Source: CAD feature listing. Evaluate the final solid. Frame: model axes, mm. A direction names the side the tool comes from. Round coordinates to 2 decimals unless told otherwise and drop trailing zeros. Order: outer loops, then holes, each group sorted by start corner. A loop starts at its lowest first (then second) coordinate and runs counter-clockwise, first axis right, second up. Notation, with made-up numbers: M -37.75,16 L 3.25,16 A25 cw 3.25,30 Z; hole C -9.5,53.5 d5. An arc over 180 degrees is marked long. Use one line per item in the form item = value. Start each with the question number.
Q1. Reachability of faces 1 (the flat face through (40.488, 0, -4)), 2 (the cylindrical face through (32.51, 9.78, 3.08)), 3 (the cylindrical face through (3.8, -1.72, -7.75)), 4 (the cylindrical face through (11.52, -1.71, -7.72)) from +Z, -Z, +X, -X, +Y, -Y: full face, straight path, thin tool, end or side. Return the list, or none.
Q2. Section B-B (y = 0). Give the number of separate pieces and of enclosed holes in the cut face, plus the area to 3 significant figures.
Q3. Pull-direction query (Z, two-part tool) for faces 5 (the cylindrical face through (34.648, -1.931, -8.697)), 6 (the cylindrical face through (8.797, 6.523, 2.054)), 7 (the conical face through (19.68, 0.06, 10.43)); classes: pulls with the +Z half, pulls with the -Z half, needs draft (parallel to the pull), parting line crosses it, or undercut.
Q4. Contact query for flat-ended pins moving along their axis: pin 1 (10 mm diameter, centred on y = -8, z = 0.5, fed in from -X); pin 2 (12 mm diameter, centred on x = 25, y = 7.5, fed in from +Z); pin 3 (10 mm diameter, centred on x = 24.61, y = 0, fed in from +Z); pin 4 (2 mm diameter, centred on y = 7, z = 5.5, fed in from -X). Output: stop coordinate, or through.
Q5. Section A-A (x = 9). Return the cut outline in (y, z).
Q6. Material intervals for probe 1 along Z at (x, y) = (11.5, 0); probe 2 along X at (y, z) = (7.5, 3.5); probe 3 along Z at (x, y) = (14.5, 0), sorted ascending.
Autodesk Inventor part; units mm, degrees
ref_plane "s1_XY" through (10.3124, 0, 0) normal (0, 0, 1) x (1, 0, 0)
ref_plane "s1_YZ" through (10.3124, 0, 0) normal (1, 0, 0) x (0, 1, 0)
ref_plane "s1_ZX" through (10.3124, 0, 0) normal (0, 1, 0) x (0, 0, 1)
sketch "Sketch_2" plane through (0, 0, 0) normal (0, 0, 1) x (1, 0, 0)
  line L0 (12.7, 0) -> (0, 0)
  line L1 (0, 0) -> (0, 7.098)
  line L2 (0, 7.098) -> (0.8395, 7.9375)
  line L3 (0.8395, 7.9375) -> (6.6816, 7.9375)
  line L4 (6.6816, 7.9375) -> (7.5223, 7.0968)
  arc A0 (7.5223, 7.0968) -> (8.1407, 6.839) centre (8.1385, 7.7041) ccw
  line L5 (8.1407, 6.839) -> (9.4361, 6.839)
  arc A1 (9.4361, 6.839) -> (10.3124, 7.7153) centre (9.4361, 7.7152) ccw
  line L6 (10.3124, 7.7153) -> (10.3124, 7.9057)
  line L7 (10.3124, 7.9057) -> (12.7, 7.9057)
  line L8 (12.7, 7.9057) -> (12.7, 0)
  line L9 (12.7, 0) -> (0, 0)
revolve "Revolution1" add sketch "Sketch_2" angle 360 about axis through (12.7, 0, 0) along (1, 0, 0)
thread "Thread1"
sketch "Sketch_3" plane through (0, 0, 0) normal (0, 0, 1) x (1, 0, 0)
  line L0 (40.4876, 0) -> (12.7, 0)
  line L1 (12.7, 0) -> (12.7, 10.1918)
  line L2 (12.7, 10.1918) -> (13.462, 10.9537)
  line L3 (13.462, 10.9537) -> (34.0741, 10.9537)
  line L4 (34.0741, 10.9537) -> (34.0741, 8.9091)
  line L5 (34.0741, 8.9091) -> (34.8361, 8.9091)
  line L6 (34.8361, 8.9091) -> (35.5981, 9.671)
  line L7 (35.5981, 9.671) -> (39.7256, 9.671)
  line L8 (39.7256, 9.671) -> (40.4876, 8.9091)
  line L9 (40.4876, 8.9091) -> (40.4876, 0)
  line L10 (40.4876, 0) -> (12.7, 0)
revolve "Revolution2" add sketch "Sketch_3" angle 360 about axis through (40.4876, 0, 0) along (1, 0, 0)
sketch "Sketch3" plane through (0, 0, 0) normal (-1, 0, 0) x (0, 0, 1)
  point P0 (0, 0)
hole "Drilling 1" at (0, 0, 0) direction (1, 0, 0) diameter 6.4389 depth 40.4876 countersink diameter 6.9469 countersink angle 90
sketch "Sketch_10" plane through (0, 0, 0) normal (0, 0, 1) x (1, 0, 0)
  line L0 (34.0741, 0) -> (30.8991, 0)
  line L1 (30.8991, 10.2553) -> (34.0741, 10.2553)
  line L2 (34.0741, 10.2553) -> (34.0741, 15.3353)
  line L3 (34.0741, 15.3353) -> (30.8991, 15.3353)
  line L4 (30.8991, 15.3353) -> (30.8991, 10.2553)
revolve "Revolution3" cut sketch "Sketch_10" angle 360 about axis through (34.0741, 0, 0) along (1, 0, 0)
sketch "Sketch_40" plane through (0, 0, 0) normal (0, 1, 0) x (-1, 0, 0)
  line L0 (-24.6126, 10.9537) -> (-24.6126, 0)
  line L1 (-24.6126, 0) -> (-27.7876, 0)
  line L2 (-27.7876, 0) -> (-27.7876, 3.7572)
  line L3 (-27.7876, 3.7572) -> (-29.2538, 4.6037)
  line L4 (-29.2538, 4.6037) -> (-29.4323, 10.3187)
  line L5 (-29.4323, 10.3187) -> (-30.0673, 10.9537)
  line L6 (-30.0673, 10.9537) -> (-24.6126, 10.9537)
  line L7 (-24.6126, 10.9537) -> (-24.6126, 0)
revolve "Revolution4" cut sketch "Sketch_40" angle 360 about axis through (24.6126, 0, 10.9537) along (0, 0, 1)
thread "Thread2"
sketch "Sketch_47" plane through (0, 0, 0) normal (0, 0, 1) x (1, 0, 0)
  line L0 (34.8361, 0) -> (34.0741, 0)
  line L1 (34.0741, 8.655) -> (34.8361, 8.655)
  line L2 (34.8361, 8.655) -> (34.8361, 8.9091)
  line L3 (34.8361, 8.9091) -> (34.4551, 8.9091)
  line L4 (34.4551, 8.9091) -> (34.1966, 9.1676)
  arc A0 (34.1966, 9.3472) -> (34.1966, 9.1676) centre (34.2864, 9.2574) ccw
  line L5 (34.1966, 9.3472) -> (35.0205, 10.1711)
  line L6 (35.0205, 10.1711) -> (35.0205, 10.2553)
  line L7 (35.0205, 10.2553) -> (34.8173, 10.2553)
  line L8 (34.8173, 10.2553) -> (34.0741, 9.512)
  line L9 (34.0741, 9.512) -> (34.0741, 8.655)
revolve "Revolution5" add sketch "Sketch_47" angle 360 about axis through (34.8361, 0, 0) along (1, 0, 0)
ref_plane "s1_XY" through (10.3124, 0, 0) normal (0, 0, 1) x (1, 0, 0)
ref_plane "s1_YZ" through (10.3124, 0, 0) normal (1, 0, 0) x (0, 1, 0)
ref_plane "s1_ZX" through (10.3124, 0, 0) normal (0, 1, 0) x (0, 0, 1)
ref_plane "s2_XY" through (12.7, 0, 0) normal (0, 0, 1) x (1, 0, 0)
ref_plane "s2_YZ" through (12.7, 0, 0) normal (1, 0, 0) x (0, 1, 0)
ref_plane "s2_ZX" through (12.7, 0, 0) normal (0, 1, 0) x (0, 0, 1)
ref_plane "dp1_XY" through (12.7, 7.9057, 0) normal (0, 0, 1) x (1, 0, 0)
ref_plane "dp1_YZ" through (12.7, 7.9057, 0) normal (1, 0, 0) x (0, 1, 0)
ref_plane "dp1_ZX" through (12.7, 7.9057, 0) normal (0, 1, 0) x (0, 0, 1)
ref_plane "dp2_XY" through (12.7, -7.9057, 0) normal (0, 0, 1) x (1, 0, 0)
ref_plane "dp2_YZ" through (12.7, -7.9057, 0) normal (1, 0, 0) x (0, 1, 0)
ref_plane "dp2_ZX" through (12.7, -7.9057, 0) normal (0, 1, 0) x (0, 0, 1)
ref_plane "rod_guide_XY" through (0, 0, 0) normal (1, 0, 0) x (0, 0, -1)
ref_plane "rod_guide_YZ" through (0, 0, 0) normal (0, 0, -1) x (0, 1, 0)
ref_plane "rod_guide_ZX" through (0, 0, 0) normal (0, 1, 0) x (1, 0, 0)
ref_plane "to_tube_XY" through (34.8361, 0, 0) normal (1, 0, 0) x (0, 0, -1)
ref_plane "to_tube_YZ" through (34.8361, 0, 0) normal (0, 0, -1) x (0, 1, 0)
ref_plane "to_tube_ZX" through (34.8361, 0, 0) normal (0, 1, 0) x (1, 0, 0)
ref_plane "to_foot_bracket_XY" through (12.7, 0, 0) normal (1, 0, 0) x (0, 0, -1)
ref_plane "to_foot_bracket_YZ" through (12.7, 0, 0) normal (0, 0, -1) x (0, 1, 0)
ref_plane "to_foot_bracket_ZX" through (12.7, 0, 0) normal (0, 1, 0) x (1, 0, 0)
ref_plane "to_nut_XY" through (10.3124, 0, 0) normal (1, 0, 0) x (0, 0, -1)
ref_plane "to_nut_YZ" through (10.3124, 0, 0) normal (0, 0, -1) x (0, 1, 0)
ref_plane "to_nut_ZX" through (10.3124, 0, 0) normal (0, 1, 0) x (1, 0, 0)
ref_plane "to_trunnion_brackets_XY" through (11.1252, 0, 0) normal (0, 1, 0) x (1, 0, 0)
ref_plane "to_trunnion_brackets_YZ" through (11.1252, 0, 0) normal (1, 0, 0) x (0, 0, -1)
ref_plane "to_trunnion_brackets_ZX" through (11.1252, 0, 0) normal (0, 0, -1) x (0, 1, 0)
ref_plane "to_trunnion_brackets1_XY" through (11.1252, 12.7, 0) normal (0, 1, 0) x (1, 0, 0)
ref_plane "to_trunnion_brackets1_YZ" through (11.1252, 12.7, 0) normal (1, 0, 0) x (0, 0, -1)
ref_plane "to_trunnion_brackets1_ZX" through (11.1252, 12.7, 0) normal (0, 0, -1) x (0, 1, 0)
ref_plane "to_trunnion_brackets2_XY" through (11.1252, -12.7, 0) normal (0, 1, 0) x (1, 0, 0)
ref_plane "to_trunnion_brackets2_YZ" through (11.1252, -12.7, 0) normal (1, 0, 0) x (0, 0, -1)
ref_plane "to_trunnion_brackets2_ZX" through (11.1252, -12.7, 0) normal (0, 0, -1) x (0, 1, 0)
ref_plane "t111_XY" through (12.7, 0, 0) normal (1, 0, 0) x (0, 0, -1)
ref_plane "t111_YZ" through (12.7, 0, 0) normal (0, 0, -1) x (0, 1, 0)
ref_plane "t111_ZX" through (12.7, 0, 0) normal (0, 1, 0) x (1, 0, 0)
ref_plane "t1_XY" through (12.7, 0, 0) normal (1, 0, 0) x (0, 0, -1)
ref_plane "t1_YZ" through (12.7, 0, 0) normal (0, 0, -1) x (0, 1, 0)
ref_plane "t1_ZX" through (12.7, 0, 0) normal (0, 1, 0) x (1, 0, 0)
ref_plane "port_XY" through (24.6126, 0, 0) normal (0, 0, 1) x (1, 0, 0)
ref_plane "port_YZ" through (24.6126, 0, 0) normal (1, 0, 0) x (0, 1, 0)
ref_plane "port_ZX" through (24.6126, 0, 0) normal (0, 1, 0) x (0, 0, 1)
ref_plane "to_screw_XY" through (24.6126, 2.032, -6.0452) normal (0, 1, 0) x (1, 0, 0)
ref_plane "to_screw_YZ" through (24.6126, 2.032, -6.0452) normal (1, 0, 0) x (0, 0, -1)
ref_plane "to_screw_ZX" through (24.6126, 2.032, -6.0452) normal (0, 0, -1) x (0, 1, 0)
properties part number "04R000_rod_guide"
Results list:
q1.face_1 = +Z, -Z, +X, +Y, -Y
q1.face_2 = +X
q1.face_3 = -X
q1.face_4 = none
q2.separate_pieces = 3
q2.enclosed_holes = 0
q2.area = 449 mm2
q3.face_5 = undercut
q3.face_6 = parting line crosses it
q3.face_7 = pulls with the +Z half
q4.pin_1 = 0
q4.pin_2 = 10.57
q4.pin_3 = 10.5
q4.pin_4 = 0.8
q5.outline = C 0,0 d13.68; hole C 0,0 d6.44
q6.probe_1 = -7.91 to -3.22, 3.22 to 7.91
q6.probe_2 = 12.7 to 40.49
q6.probe_3 = -10.95 to -3.22, 3.22 to 10.95
